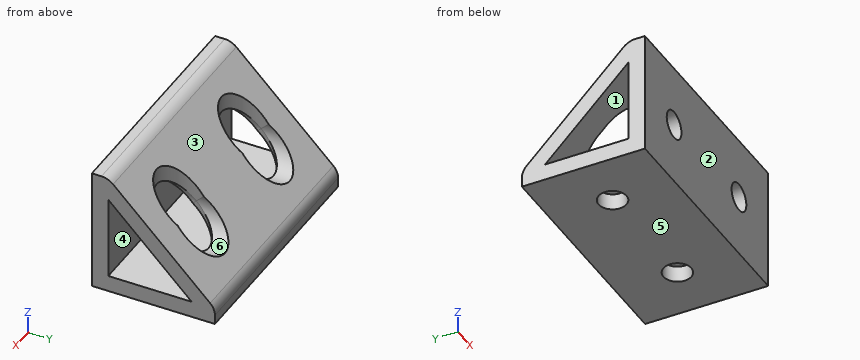
Autodesk Inventor part; units mm, degrees
ref_plane "YZ Plane" through (0, 0, 0) normal (1, 0, 0) x (0, 1, 0)
ref_plane "XZ Plane" through (0, 0, 0) normal (0, 1, 0) x (-1, 0, 0)
ref_plane "XY Plane" through (0, 0, 0) normal (0, 0, 1) x (1, 0, 0)
sketch "Sketch_1" plane through (0, 0, 0) normal (1, 0, 0) x (0, 1, 0)
  line L0 (2.3431, 30) -> (0, 30)
  line L1 (0, 30) -> (0, 0)
  line L2 (0, 0) -> (30, 0)
  line L3 (30, 0) -> (30, 2.3431)
  arc A0 (30, 2.3431) -> (28.8284, 5.1716) centre (26, 2.3431) ccw
  line L4 (28.8284, 5.1716) -> (5.1716, 28.8284)
  arc A1 (5.1716, 28.8284) -> (2.3431, 30) centre (2.3431, 26) ccw
  line L5 (4, 24.3431) -> (4, 4)
  line L6 (4, 4) -> (24.3431, 4)
  line L7 (24.3431, 4) -> (4, 24.3431)
extrude "Extrusion1" add sketch "Sketch_1" along normal mid plane 57
sketch "Sketch2" plane through (-28.5, 0, 0) normal (0, -1, 0) x (1, 0, 0)
  point P0 (43.5, 15)
hole "Hole1" at (15, 0, 15) direction (0, 1, 0) diameter 6.81 depth 4
sketch "Sketch3" plane through (28.5, 30, 0) normal (0, 0, -1) x (-1, 0, 0)
  point P0 (13.5, -15)
hole "Hole2" at (15, 15, 0) direction (0, 0, 1) diameter 6.81 depth 4
sketch "Sketch_4" plane through (0, 0, 30) normal (0, 0, 1) x (1, 0, 0)
  circle A0 centre (15, 15) radius 6.35
extrude "Extrusion2" cut sketch "Sketch_4" against normal blind 26
sketch "Sketch_5" plane through (0, 30, 0) normal (0, 1, 0) x (1, 0, 0)
  circle A0 centre (15, -15) radius 6.35
extrude "Extrusion3" cut sketch "Sketch_5" against normal blind 26
sketch "Sketch6" plane through (28.5, 30, 0) normal (0, 0, -1) x (-1, 0, 0)
  point P0 (43.5, -15)
hole "Hole3" at (-15, 15, 0) direction (0, 0, 1) diameter 6.81 depth 4
sketch "Sketch7" plane through (-28.5, 0, 0) normal (0, -1, 0) x (1, 0, 0)
  point P0 (13.5, 15)
hole "Hole4" at (-15, 0, 15) direction (0, 1, 0) diameter 6.81 depth 4
sketch "Sketch_8" plane through (0, 30, 0) normal (0, 1, 0) x (1, 0, 0)
  circle A0 centre (-15, -15) radius 6.35
extrude "Extrusion4" cut sketch "Sketch_8" against normal blind 26
sketch "Sketch_9" plane through (0, 0, 30) normal (0, 0, 1) x (1, 0, 0)
  circle A0 centre (-15, 15) radius 6.35
extrude "Extrusion5" cut sketch "Sketch_9" against normal blind 26
properties part number "30-4134 Aluminum"
Source: CAD feature listing. Evaluate the final solid. Frame: model axes, mm. Face numbers are marked on the shaded views. A direction names the side the tool comes from. Give positions to 0.01 mm unless a question says otherwise; leave off trailing zeros. Write each loop counter-clockwise with the first axis right and the second up, starting at its lowest first coordinate (ties: lowest second). Pieces come first, ordered by that corner, then holes.
1. Section query A-A (x = -15). Return the cut outline in (y, z) (3 decimals).
2. Pull-direction query (Z, two-part tool) for the marked faces 1, 2 and 3; classes: +Z half, -Z half, draft (parallel to the pull), parting line (faces both ways), or undercut.
3. Material intervals for line 1 along X through (y, z) = (15, 0.8) (3 decimals); line 2 along X through (y, z) = (13.75, 1.5); line 3 along Z through (x, y) = (-20, 20.5), sorted ascending.
4. Section query C-C (y = 10.5). Return the cut outline in (x, z).
5. Access query for the marked faces 4, 5 and 6. Directions: +Z, -Z, +X, -X, +Y, -Y. A direction counts if a zero-diameter tool reaches every point of the face in a straight line with its end or side. Return the directions, or none.
6. Section query B-B (z = 20). Return the cut outline in (x, y), then the cut area to 3 significant figures.
7. Section query D-D (y = 16.25). Count the separate pieces of the cut face and the enclosed holes in it, then the cut area to 3 significant figures.
8. First-contact query: pin 1 (4 mm diameter, centred on y = 19, z = 20, fed in from -X); pin 2 (8 mm diameter, centred on x = 16.5, y = 13.5, fed in from +Z); pin 3 (16.5 mm diameter, centred on x = 15, z = 15, fed in from +Y); pin 4 (4 mm diameter, centred on x = -9.5, z = 21, fed in from +Y). Flat tips, straight axial feed; report the tip coordinate or a pass-through.
Output values:
1. outline: (0, 0) - (11.595, 0) - (11.595, 4) - (4, 4) - (4, 11.595) - (0, 11.595) - close; (0, 18.405) - (4, 18.405) - (4, 24.343) - (6.993, 21.35) - (8.65, 21.35) - (8.65, 25.35) - (5.172, 28.828) arc R4 ccw to (2.343, 30) - (0, 30) - close; (18.405, 0) - (30, 0) - (30, 2.343) arc R4 ccw to (28.828, 5.172) - (25.35, 8.65) - (21.35, 8.65) - (21.35, 6.993) - (24.343, 4) - (18.405, 4) - close
2. face 1: undercut
2. face 2: draft
2. face 3: +Z half
3. line 1: x = -28.5 to -18.405, -11.595 to 11.595, 18.405 to 28.5
3. line 2: x = -28.5 to -18.17, -11.83 to 11.83, 18.17 to 28.5
3. line 3: z = 0 to 4, 7.84 to 11.09
4. outline: (-28.5, 0) - (28.5, 0) - (28.5, 4) - (-28.5, 4) - close; (-28.5, 17.84) - (-20.68, 17.84) arc R6.35 cw to (-19.48, 19.5) - (-19.48, 23.5) - (-28.5, 23.5) - close; (-10.52, 19.5) arc R6.35 cw to (-9.32, 17.84) - (9.32, 17.84) arc R6.35 cw to (10.52, 19.5) - (10.52, 23.5) - (-10.52, 23.5) - close; (19.48, 19.5) arc R6.35 cw to (20.68, 17.84) - (28.5, 17.84) - (28.5, 23.5) - (19.48, 23.5) - close
5. face 4: +X, -X
5. face 5: -Z, +X, -X, +Y, -Y
5. face 6: +Y
6. outline: (-28.5, 0) - (28.5, 0) - (28.5, 4) - (-28.5, 4) - close; (-28.5, 8.34) - (-18.91, 8.34) - (-18.91, 10) arc R6.35 cw to (-21.27, 14) - (-28.5, 14) - close; (-11.09, 8.34) - (11.09, 8.34) - (11.09, 10) arc R6.35 cw to (8.73, 14) - (-8.73, 14) arc R6.35 cw to (-11.09, 10) - close; (18.91, 8.34) - (28.5, 8.34) - (28.5, 14) - (21.27, 14) arc R6.35 cw to (18.91, 10) - close
6. area: 438 mm2
7. separate pieces: 6
7. enclosed holes: 0
7. area: 358 mm2
8. pin 1: passes through
8. pin 2: stops at z = 4
8. pin 3: stops at y = 27.25
8. pin 4: stops at y = 14.81
